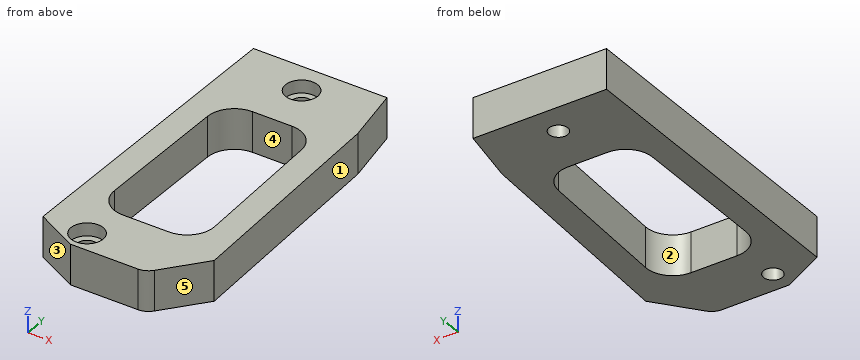
```python
from build123d import *

# Parameters (mm, degrees)
F1_DEPTH = 7.5
F3_DEPTH = 7.5
F4_R     = 1.75
F5_DEPTH = 7.5
F6_R     = 3
F7_DEPTH = 2.4
F8_R     = 3
F9_R     = 5
F10_R    = 5
F11_R    = 5
F12_R    = 5


with BuildPart() as f1:
    # F0 (on Top) → F1 (new body)
    with BuildSketch(Plane.XY):
        Polygon((7.046259, 38.376067), (-17.953741, 38.376067), (-17.953741, -19.623933), (-9.953741, -23.773933), (4.046259, -23.773933), (11.046259, -15.123933), (9.046259, 27.376067), align=None)
    extrude(amount=F1_DEPTH)

    # F2 (on face) → F3 (cut, through all)
    with BuildSketch(Plane.XY.offset(7.5)):
        Polygon((4.228961, 23.376067), (-12.953741, 23.376067), (-12.953741, -12.323933), (5.908961, -12.323933), align=None)
    extrude(amount=-F3_DEPTH, mode=Mode.SUBTRACT)

    # F4 (on face) → F5 (cut, through all)
    with BuildSketch(Plane.XY.offset(7.5)):
        with Locations((-5.053741, 32.646067)):
            Circle(F4_R)
        with Locations((-9.603741, -19.773933)):
            Circle(F4_R)
    extrude(amount=-F5_DEPTH, mode=Mode.SUBTRACT)

    # F6 (on face) → F7 (cut)
    with BuildSketch(Plane.XY.offset(7.5)):
        with Locations((-5.053741, 32.646067)):
            Circle(F6_R)
        with Locations((-9.603741, -19.773933)):
            Circle(F6_R)
    extrude(amount=-F7_DEPTH, mode=Mode.SUBTRACT)

    # F8
    f8_edges = [f1.edges().sort_by_distance(p)[0] for p in [
        (4.046259, -23.773933, 3.75),
    ]]
    fillet(f8_edges, radius=F8_R)

    # F9
    f9_edges = [f1.edges().sort_by_distance(p)[0] for p in [
        (-12.953741, -12.323933, 3.75),
    ]]
    fillet(f9_edges, radius=F9_R)

    # F10
    f10_edges = [f1.edges().sort_by_distance(p)[0] for p in [
        (5.908961, -12.323933, 3.75),
    ]]
    fillet(f10_edges, radius=F10_R)

    # F11
    f11_edges = [f1.edges().sort_by_distance(p)[0] for p in [
        (-12.953741, 23.376067, 3.75),
    ]]
    fillet(f11_edges, radius=F11_R)

    # F12
    f12_edges = [f1.edges().sort_by_distance(p)[0] for p in [
        (4.228961, 23.376067, 3.75),
    ]]
    fillet(f12_edges, radius=F12_R)


solid = f1.part
```
Source: CAD feature listing. Evaluate the final solid. Frame: model axes, mm. Face numbers are marked on the shaded views. A direction names the side the tool comes from. Round coordinates to 2 decimals unless told otherwise and drop trailing zeros. Loops run counter-clockwise (first coordinate to the right, second up) from the corner with the lowest first, then second, coordinate; pieces in that order, holes last. Notation, with made-up numbers: M 50.5,-33.75 L 56.5,-33.75 A28 ccw 56.5,-10.75 Z; hole C -25,60.25 d3. An arc over 180 degrees is marked long. Use a Markdown table: item, result. Add a question column.
1. Cut plane D-D, the plane y = 6. Output: boundary loops of the cut face in (x, z).
2. Cut plane B-B, the plane z = 2.25. Output: boundary loops of the cut face in (x, y), and give its area (3 significant figures).
3. Contact query for flat-ended pins moving along their axis: pin 1 (1 mm diameter, centred on x = -11, z = 1, fed in from -Y); pin 2 (1 mm diameter, centred on x = -12.5, z = 4.5, fed in from -Y); pin 3 (4 mm diameter, centred on y = 10.5, z = 3.5, fed in from +X). Output: stop coordinate, or through.
4. Pull-direction query (X, two-part tool) for the marked faces 3, 4 and 5; classes: +X half, -X half, draft (parallel to the pull), parting line (faces both ways), or undercut.
5. Set-up query: the marked faces 1 and 2. Return all of +Z, -Z, +X, -X, +Y, -Y with unobstructed straight access to the full face (end or side cutting, diameter ignored); none if empty.
6. Cut plane C-C, the plane x = -4. Output: boundary loops of the cut face in (y, z), and give its area (3 significant figures).
7. Cut plane A-A, the plane y = -9. Output: boundary loops of the cut face in (x, z), and give its area (3 significant figures).
8. Ray query, line 1 along Y through (x, z) = (-10.5, 2.75); line 2 along Y through (x, z) = (-0.25, 6); line 3 along X through (y, z) = (22, 6.5). Return the intervals inside material, ascending. Write a range as [from, to].
Solution:
| question | item | result |
|---|---|---|
| 1 | outline | M -17.95,0 L -12.95,0 L -12.95,7.5 L -17.95,7.5 Z; M 5.05,0 L 10.05,0 L 10.05,7.5 L 5.05,7.5 Z |
| 2 | outline | M -17.95,-19.62 L -9.95,-23.77 L 2.61,-23.77 A3 ccw 4.95,-22.66 L 11.05,-15.12 L 9.05,27.38 L 7.05,38.38 L -17.95,38.38 Z; hole M -12.95,-7.32 A5 ccw -7.95,-12.32 L 0.67,-12.32 A5 ccw 5.66,-7.09 L 4.45,18.61 A5 ccw -0.54,23.38 L -7.95,23.38 A5 ccw -12.95,18.38 Z; hole C -9.6,-19.77 d3.5; hole C -5.05,32.65 d3.5 |
| 2 | area | 1,040 mm2 |
| 3 | pin 1 | stops at y = -23.49 |
| 3 | pin 2 | stops at y = -22.71 |
| 3 | pin 3 | stops at x = 9.93 |
| 4 | face 3 | -X half |
| 4 | face 4 | undercut |
| 4 | face 5 | +X half |
| 5 | face 1 | +Z, -Z, +X, +Y |
| 5 | face 2 | +Z, -Z |
| 6 | outline | M -23.77,0 L -12.32,0 L -12.32,7.5 L -23.77,7.5 Z; M 23.38,0 L 31.25,0 L 31.25,5.1 L 29.84,5.1 L 29.84,7.5 L 23.38,7.5 Z; M 34.04,0 L 38.38,0 L 38.38,7.5 L 35.45,7.5 L 35.45,5.1 L 34.04,5.1 Z |
| 6 | area | 171 mm2 |
| 7 | outline | M -17.95,0 L -12.66,0 L -12.66,7.5 L -17.95,7.5 Z; M 5.38,0 L 10.76,0 L 10.76,7.5 L 5.38,7.5 Z |
| 7 | area | 80.0 mm2 |
| 8 | line 1 | y = [-23.49, -21.28], [-18.27, -11.63], [22.68, 38.38] |
| 8 | line 2 | y = [-23.77, -12.32], [23.37, 38.38] |
| 8 | line 3 | x = [-17.95, -11.4], [2.9, 9.3] |
